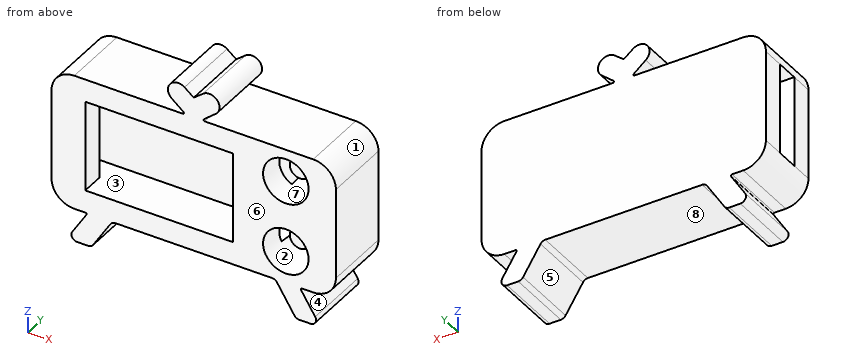
```python
from build123d import *

# Parameters (mm, degrees)
F3_DEPTH  = 30
F4_W      = 20
F4_H      = 80
F5_DEPTH  = 199
F6_R      = 20
F7_DEPTH  = 40
F7_TAPER  = 5
F0_W      = 130
F0_H      = 80
F8_DEPTH  = 43
F9_R      = 9
F10_DEPTH = 20


with BuildPart() as f3:
    # F2 (on Front) → F3 (new body, symmetric)
    with BuildSketch(Plane.XZ):
        with BuildLine():
            ThreePointArc((-94.639390707, -40), (-88.7815263307, -54.1421356237), (-74.639390707, -60))
            Line((-74.639390707, -60), (-64.7730480564, -60))
            ThreePointArc((-64.7730480564, -60), (-63.8977460335, -60.5164233581), (-63.9264968306, -61.5323072629))
            Line((-63.9264968306, -61.5323072629), (-76.4204092514, -81.4019156883))
            ThreePointArc((-76.4204092514, -81.4019156883), (-76.5641632373, -86.481335212), (-72.1876531224, -89.0634520026))
            Line((-72.1876531224, -89.0634520026), (-62.3831424536, -89.0634520026))
            ThreePointArc((-62.3831424536, -89.0634520026), (-59.9652592442, -88.4399621175), (-58.1503863246, -86.7249883169))
            Line((-58.1503863246, -86.7249883169), (-42.8162591257, -62.3384636857))
            ThreePointArc((-42.8162591257, -62.3384636857), (-41.0013862061, -60.6234898851), (-38.5835029967, -60))
            Line((-38.5835029967, -60), (99.3047215826, -60))
            ThreePointArc((99.3047215826, -60), (101.7226047921, -60.6234898851), (103.5374777117, -62.3384636857))
            Line((103.5374777117, -62.3384636857), (118.8716049106, -86.7249883169))
            ThreePointArc((118.8716049106, -86.7249883169), (120.6864778302, -88.4399621175), (123.1043610396, -89.0634520026))
            Line((123.1043610396, -89.0634520026), (132.9088717083, -89.0634520026))
            ThreePointArc((132.9088717083, -89.0634520026), (137.2853818232, -86.481335212), (137.1416278374, -81.4019156883))
            Line((137.1416278374, -81.4019156883), (124.6477154166, -61.5323072629))
            ThreePointArc((124.6477154166, -61.5323072629), (124.6189646194, -60.5164233581), (125.4942666424, -60))
            Line((125.4942666424, -60), (135.360609293, -60))
            ThreePointArc((135.360609293, -60), (149.5027449167, -54.1421356237), (155.360609293, -40))
            Line((155.360609293, -40), (155.360609293, 40))
            ThreePointArc((155.360609293, 40), (149.5027449167, 54.1421356237), (135.360609293, 60))
            Line((135.360609293, 60), (39.9569445726, 60))
            ThreePointArc((39.9569445726, 60), (39.0153160887, 60.6633461743), (39.3229389096, 61.7733284033))
            Line((39.3229389096, 61.7733284033), (49.6255289763, 70.2198052406))
            ThreePointArc((49.6255289763, 70.2198052406), (51.1272936037, 82.8727111049), (38.4743877395, 84.3744757323))
            Line((38.4743877395, 84.3744757323), (30.360609293, 77.9823884368))
            Line((30.360609293, 77.9823884368), (22.2468308465, 84.3744757323))
            ThreePointArc((22.2468308465, 84.3744757323), (9.5939249823, 82.8727111049), (11.0956896096, 70.2198052406))
            Line((11.0956896096, 70.2198052406), (21.3982796764, 61.7733284033))
            ThreePointArc((21.3982796764, 61.7733284033), (21.7059024972, 60.6633461743), (20.7642740134, 60))
            Line((20.7642740134, 60), (-74.639390707, 60))
            ThreePointArc((-74.639390707, 60), (-88.7815263307, 54.1421356237), (-94.639390707, 40))
            Line((-94.639390707, 40), (-94.639390707, -40))
        make_face()
    extrude(amount=F3_DEPTH, both=True)

    # F4 (on face) → F5 (cut)
    with BuildSketch(Plane(origin=(-94.639390707, 0, 0), x_dir=(0, -1, 0), z_dir=(-1, 0, 0))):
        Rectangle(F4_W, F4_H)
    extrude(amount=-F5_DEPTH, mode=Mode.SUBTRACT)

    # F6 (on face) → F7 (cut)
    with BuildSketch(Plane.XZ.offset(30)):
        with Locations((111.3148257136, 31.6125191748)):
            Circle(F6_R)
        with Locations((111.3148257136, -31.6125191748)):
            Circle(F6_R)
    extrude(amount=-F7_DEPTH, taper=F7_TAPER, mode=Mode.SUBTRACT)

    # F0 (on Front) → F8 (cut)
    with BuildSketch(Plane.XZ):
        Rectangle(F0_W, F0_H)
    extrude(amount=F8_DEPTH, mode=Mode.SUBTRACT)

    # F9 (on face) → F10 (join)
    with BuildSketch(Plane.XZ.offset(-10)):
        with Locations((111.3148257136, 31.6125191748)):
            Circle(F9_R)
        with Locations((111.3148257136, -31.6125191748)):
            Circle(F9_R)
    extrude(amount=F10_DEPTH)


solid = f3.part
```
Model file for the job. Use its own axes, mm. Face numbers are marked on the shaded views. A direction names the side the tool comes from. Give positions to 0.01 mm unless a question says otherwise; leave off trailing zeros. Write each loop counter-clockwise with the first axis right and the second up, starting at its lowest first coordinate (ties: lowest second). Pieces come first, ordered by that corner, then holes. Notation, with made-up numbers: (8.25, 80.25) -> (65.25, 80.25) arc R21 ccw to (65.25, 96.25) -> close; hole circle Ø5 at (59.25, -28.75). An arc over 180 degrees is marked (long way). Use CSV: the item, a comma, the result in double quotes. Start each with the question number.
1) Tool access for the marked faces 1, 2, 3, 4 and 5: list every direction of +Z, -Z, +X, -X, +Y, -Y with a clear straight run to the whole face (end or side of a thin tool).
2) Cut at A-A on z = -9. List the corners of the cut face in (x, y), plus the area to 3 significant figures.
3) Pin check, flat tips, straight feed: P1, Ø9, axis at x = 111.5, z = -29, coming from the -Y side; P2, Ø20, axis at x = 6, y = -16.5, coming from the +Z side; P3, Ø12, axis at y = 9, z = -55.5, coming from the -X side. Stop position of each tip, or through.
4) Two-plate mould, pull along Z, no slides. Class the marked faces 6, 7 and 8: released by +Z, released by -Z, zero draft, split by the parting line, or undercut.
5) Drill centre lines: L1, parallel to Z at x = 96.5, y = 9; L2, parallel to X at y = -13.5, z = -7; L3, parallel to Z at x = 12.5, y = -1. Where is each one in solid material? Low to high.
6) Cut at C-C on x = -14.5. List the corners of the cut face in (y, z), plus the area to 3 significant figures.
7) Cut at B-B on x = 70. List the corners of the cut face in (y, z).
Final values:
1,face 1,"+Z, +X, +Y, -Y"
1,face 2,"-Y"
1,face 3,"none"
1,face 4,"+X, +Y, -Y"
1,face 5,"-Z, +Y, -Y"
2,outline,"(-94.64, -30) -> (-65, -30) -> (-65, -10) -> (-94.64, -10) -> close; (-94.64, 10) -> (104.36, 10) -> (104.36, -10) -> (65, -10) -> (65, -30) -> (155.36, -30) -> (155.36, 30) -> (-94.64, 30) -> close"
2,area,"8,420 mm2"
3,P1,"stops at y = -10"
3,P2,"stops at z = 86.28"
3,P3,"stops at x = -92.24"
4,face 6,"zero draft"
4,face 7,"undercut"
4,face 8,"released by -Z"
5,L1,"z = -60 to -40, 40 to 60"
5,L2,"x = -94.64 to -65, 65 to 155.36"
5,L3,"z = -60 to -40, 40 to 60, 69.07 to 85.28"
6,outline,"(-30, -60) -> (30, -60) -> (30, 60) -> (-30, 60) -> (-30, 40) -> (10, 40) -> (10, -40) -> (-30, -40) -> close"
6,area,"4,000 mm2"
7,outline,"(-30, -60) -> (30, -60) -> (30, 60) -> (-30, 60) -> close; hole (-10, -40) -> (10, -40) -> (10, 40) -> (-10, 40) -> close"
